Work out the finished part from the listing and answer in its coordinate system (mm). Give positions to 0.01 mm unless a question says otherwise; leave off trailing zeros. Order: outer loops, then holes, each group sorted by start corner. A loop starts at its lowest first (then second) coordinate and runs counter-clockwise, first axis right, second up. Notation, with made-up numbers: (61.5, 49) - (70.5, 49) arc R14 ccw to (70.5, 53) - close; hole circle Ø5 at (-26.5, 54). An arc over 180 degrees is marked (long way). Put each result on its own line as item: value.
```python
from build123d import *

# Parameters (mm, degrees)
SKETCH1_R           = 3
BOSS_EXTRUDE1_DEPTH = 2


with BuildPart() as part:
    # Sketch1 → Boss-Extrude1 (new body)
    with BuildSketch(Plane.XY):
        with BuildLine():
            Line((-142.75, 49.5), (-142.75, -39.5))
            ThreePointArc((-142.75, -39.5), (-139.821067812, -46.571067812), (-132.75, -49.5))
            Line((-132.75, -49.5), (-67.25, -49.5))
            ThreePointArc((-67.25, -49.5), (-60.178932188, -46.571067812), (-57.25, -39.5))
            Line((-57.25, -39.5), (-57.25, -10))
            ThreePointArc((-57.25, -10), (-54.321067812, -2.928932188), (-47.25, 0))
            Line((-47.25, 0), (47.25, 0))
            ThreePointArc((47.25, 0), (54.321067812, -2.928932188), (57.25, -10))
            Line((57.25, -10), (57.25, -39.5))
            ThreePointArc((57.25, -39.5), (60.178932188, -46.571067812), (67.25, -49.5))
            Line((67.25, -49.5), (132.75, -49.5))
            ThreePointArc((132.75, -49.5), (139.821067812, -46.571067812), (142.75, -39.5))
            Line((142.75, -39.5), (142.75, 49.5))
            Line((142.75, 49.5), (-142.75, 49.5))
        make_face()
        with Locations((124.75, 30.5)):
            Circle(SKETCH1_R, mode=Mode.SUBTRACT)
        with Locations((124.75, -30.5)):
            Circle(SKETCH1_R, mode=Mode.SUBTRACT)
        with Locations((75.25, -30.5)):
            Circle(SKETCH1_R, mode=Mode.SUBTRACT)
        with Locations((75.25, 30.5)):
            Circle(SKETCH1_R, mode=Mode.SUBTRACT)
        with Locations((-75.25, -30.5)):
            Circle(SKETCH1_R, mode=Mode.SUBTRACT)
        with Locations((-75.25, 30.5)):
            Circle(SKETCH1_R, mode=Mode.SUBTRACT)
        with Locations((-124.75, 30.5)):
            Circle(SKETCH1_R, mode=Mode.SUBTRACT)
        with Locations((-124.75, -30.5)):
            Circle(SKETCH1_R, mode=Mode.SUBTRACT)
    extrude(amount=BOSS_EXTRUDE1_DEPTH)


solid = part.part
```
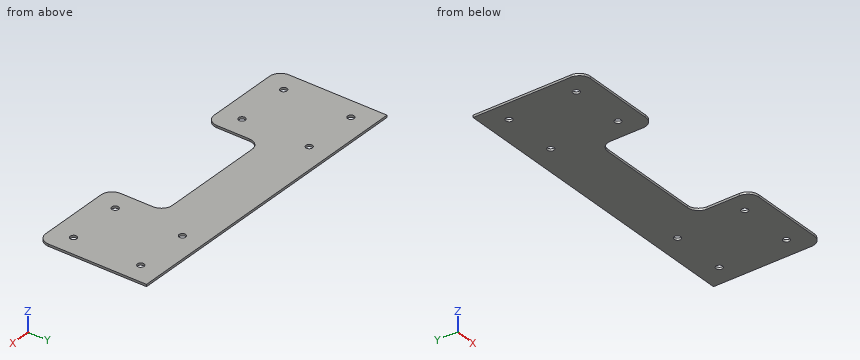
(1) Section D-D, the plane y = 30.5 is taken. Write down the section's boundary in (x, z), then the cut area to 3 significant figures.
Geometry check:
outline: (-142.75, 0) - (-127.75, 0) - (-127.75, 2) - (-142.75, 2) - close; (-121.75, 0) - (-78.25, 0) - (-78.25, 2) - (-121.75, 2) - close; (-72.25, 0) - (72.25, 0) - (72.25, 2) - (-72.25, 2) - close; (78.25, 0) - (121.75, 0) - (121.75, 2) - (78.25, 2) - close; (127.75, 0) - (142.75, 0) - (142.75, 2) - (127.75, 2) - close
area: 523 mm²
(2) Given pin 1 (5 mm diameter, centred on x = -75.25, y = 30.5, fed in from +Z); pin 2 (1 mm diameter, centred on x = -4.5, z = 1, fed in from -Y), each flat-ended and moving along its own axis, determine where each tip first touches the part or whether it passes through.
Geometry check:
pin 1: passes through
pin 2: stops at y = 0
(3) Section B-B, the plane x = -75.25 is taken. Write down the section's boundary in (y, z).
Geometry check:
outline: (-49.5, 0) - (-33.5, 0) - (-33.5, 2) - (-49.5, 2) - close; (-27.5, 0) - (27.5, 0) - (27.5, 2) - (-27.5, 2) - close; (33.5, 0) - (49.5, 0) - (49.5, 2) - (33.5, 2) - close
(4) Straight lines are drawn through the part: line 1 (Y direction, x = -75.25, z = 0.8); line 2 (X direction, y = -22, z = 0.2); line 3 (X direction, y = 32, z = 0.7). For each, find the intervals that lie inside material, in ascending order.
Geometry check:
line 1: y = -49.5 to -33.5, -27.5 to 27.5, 33.5 to 49.5
line 2: x = -142.75 to -57.25, 57.25 to 142.75
line 3: x = -142.75 to -127.35, -122.15 to -77.85, -72.65 to 72.65, 77.85 to 122.15, 127.35 to 142.75
(5) Section A-A, the plane y = -21 is taken. Write down the section's boundary in (x, z).
Geometry check:
outline: (-142.75, 0) - (-57.25, 0) - (-57.25, 2) - (-142.75, 2) - close; (57.25, 0) - (142.75, 0) - (142.75, 2) - (57.25, 2) - close
(6) Section C-C, the plane z = 0.6 is taken. Count the separate pieces of the cut face and the enclosed holes in it, then the cut area to 3 significant figures.
Geometry check:
separate pieces: 1
enclosed holes: 8
area: 22,300 mm²
